Answer from the drawing. Dimensions are ordinates in mm from the lowest x, y and z of the part. Round coordinates to 2 decimals unless told otherwise and drop trailing zeros. Order: outer loops, then holes, each group sorted by start corner. A loop starts at its lowest first (then second) coordinate and runs counter-clockwise, first axis right, second up.
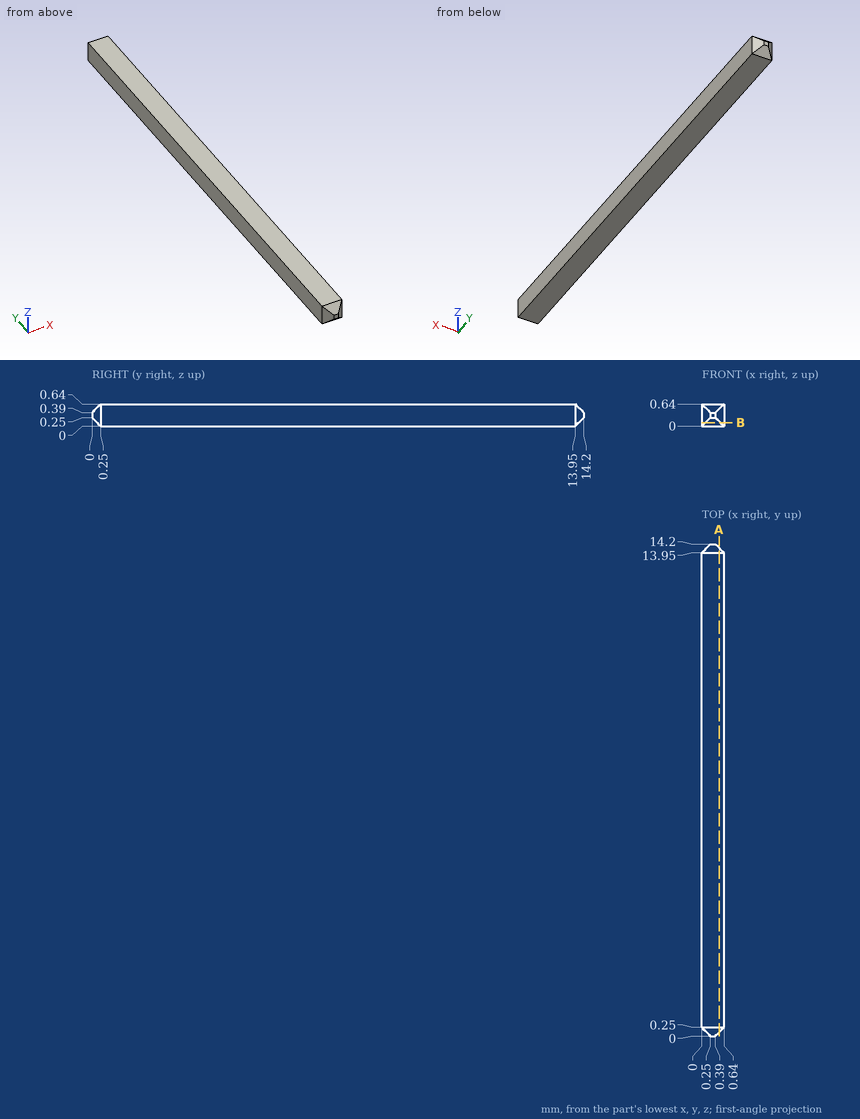
Q1. A cutting plane is placed at B-B, the plane z = 0.1. Give the vertices of the cut face in (x, y), plus the area to 3 significant figures.
Outcome:
outline: (0, 0.25) - (0.1, 0.15) - (0.54, 0.15) - (0.64, 0.25) - (0.64, 13.95) - (0.54, 14.05) - (0.1, 14.05) - (0, 13.95) - close
area: 8.88 mm2
Q2. Straight lines are drawn through the part: probe 1 along Y at (x, z) = (0.6, 0.45); probe 2 along Y at (x, z) = (0.2, 0.1). For each, find the intervals that lie inside material, in ascending order.
Outcome:
probe 1: y = 0.21 to 13.99
probe 2: y = 0.15 to 14.05
Q3. A cutting plane is placed at A-A, the plane x = 0.5. Give the vertices of the cut face in (y, z).
Outcome:
outline: (0.11, 0.14) - (0.25, 0) - (13.95, 0) - (14.09, 0.14) - (14.09, 0.5) - (13.95, 0.64) - (0.25, 0.64) - (0.11, 0.5) - close
